Verification items for the finished model (mm, model axes). A direction names the side the tool comes from. Coordinates: 2 decimals unless noted, no trailing zeros. Write each loop counter-clockwise with the first axis right and the second up, starting at its lowest first coordinate (ties: lowest second). Pieces come first, ordered by that corner, then holes. Notation, with made-up numbers: (-22, 61.25) -> (-16, 61.25) arc R24 cw to (-16, 94.25) -> close; hole circle Ø1 at (36.5, 40.25). An arc over 180 degrees is marked (long way). Use a Markdown table: item, result. Add a question column.
Autodesk Inventor part; units mm, degrees
ref_plane "YZ Plane" through (0, 0, 0) normal (1, 0, 0) x (0, 1, 0)
ref_plane "XZ Plane" through (0, 0, 0) normal (0, 1, 0) x (-1, 0, 0)
ref_plane "XY Plane" through (0, 0, 0) normal (0, 0, 1) x (1, 0, 0)
sketch "Sketch1" plane through (0, 0, 0) normal (0, 0, 1) x (1, 0, 0)
  line L0 (-110, 70) -> (110, 70) construction
  line L1 (110, 70) -> (110, -70) construction
  line L2 (110, -70) -> (-110, -70) construction
  line L3 (-110, -70) -> (-110, 70) construction
  circle A0 centre (-90, 55) radius 5
  circle A1 centre (-90, -55) radius 5
  circle A2 centre (90, -55) radius 5
  circle A3 centre (-10, 45) radius 5
  line L4 (-67, 0) -> (-42, 0) construction
  line L5 (-42, 0) -> (-42, -30) construction
  line L6 (-42, -30) -> (-67, -30) construction
  line L7 (-67, -30) -> (-67, 0) construction
  circle A4 centre (-54.5, -11) radius 10 construction
  circle A5 centre (-63.5044, -24.4163) radius 3 construction
  circle A6 centre (-57.3559, -26.4695) radius 3 construction
  circle A7 centre (-51.263, -24.6531) radius 3 construction
  circle A8 centre (-45.3418, -26.5938) radius 3 construction
  arc A9 (-75, 54.9997) -> (-105, 55) centre (-90, 55) ccw
  arc A10 (-105, -55) -> (-90, -70) centre (-90, -55) ccw
  line L8 (-105, 55) -> (-105, -55)
  line L9 (-67.173, 37.0938) -> (-15.8457, 58.814)
  arc A11 (-80.9053, 10.3283) -> (-28.4795, 28.932) centre (-131.69, 236.6113) ccw
  arc A12 (-84.9945, -37.6763) -> (-83.834, 6.647) centre (-774.2501, 2.5469) ccw
  arc A13 (-74.1138, 41.4213) -> (-75, 54.9997) centre (-774.2501, 2.5469) ccw
  arc A14 (-74.1138, 41.4213) -> (-67.173, 37.0938) centre (-69.1215, 41.6985) ccw
  arc A15 (-80.9053, 10.3283) -> (-83.834, 6.647) centre (-80.0841, 6.6693) ccw
  arc A16 (-84.9945, -37.6763) -> (-79.3208, -42.9208) centre (-80.003, -37.9675) ccw
  arc A17 (-0.2374, 33.6118) -> (-15.8457, 58.814) centre (-10, 45) ccw
  arc A18 (87.1375, -69.7243) -> (81.0789, -42.9413) centre (90, -55) ccw
  arc A19 (90, -70) -> (-90, -70) centre (0, -989.5783) ccw
  line L10 (5, 45) -> (5, -37.2895)
  arc A20 (-21.304, 23.7513) -> (-20.2259, -37.0973) centre (169.1855, -3.3075) ccw
  line L11 (-19.6904, 33.6118) -> (-19.6904, -39.9724) construction
  line L12 (-19.6904, 33.6118) -> (53.8938, 33.6118) construction
  arc A21 (-21.304, 23.7513) -> (-28.4795, 28.932) centre (-26.2543, 24.4545) ccw
  arc A22 (-22.6296, -40.0357) -> (-20.2259, -37.0973) centre (-22.687, -37.5364) ccw
  arc A23 (5, -37.2895) -> (7.4835, -39.7895) centre (7.5, -37.2895) ccw
  arc A24 (81.0789, -42.9413) -> (7.4835, -39.7895) centre (0.7495, -1057.8516) ccw
  arc A25 (-22.6296, -40.0357) -> (-79.3208, -42.9208) centre (0.7495, -1057.8516) ccw
  point P0 (0, 0)
  point P1 (90, -70)
  dimension "d1" = 70
  dimension "d2" = 70
  dimension "d3" = 110
  dimension "d4" = 110
  dimension "d5" = 10
  dimension "d6" = 10
  dimension "d7" = 10
  dimension "d8" = 10
  dimension "d9" = 55
  dimension "d10" = 55
  dimension "d11" = 55
  dimension "d12" = 180
  dimension "d13" = 90
  dimension "d14" = 90
  dimension "d15" = 10
  dimension "d16" = 45
  dimension "d17" = 42
  dimension "d18" = 30
  dimension "d19" = 0
  dimension "d20" = 25
  dimension "d21" = 20
  dimension "d22" = 6
  dimension "d23" = 6
  dimension "d24" = 6
  dimension "d25" = 11
  dimension "d26" = 12.5
  dimension "d27" = 6
  dimension "d50" = 30
  dimension "d51" = 30
  dimension "d53" = 10
  dimension "d54" = 7.5
  dimension "d58" = 10
  dimension "d59" = 30
  dimension "d60" = 30
  dimension "d61" = 90
  dimension "d62" = 10
  dimension "d63" = 5
  dimension "d64" = 5
extrude "Extrusion5" add sketch "Sketch1" along normal blind 9.4 contours A13 A14 L9 A17 L10 A23 A24 A18 A19 A10 L8 A9
equation "\"d26\" = 0.5 * d20"
properties part number "Bracket Concept MK7"
1) Gauge pin test, flat ends, axial feed: pin 1 (2 mm diameter, centred on x = -44, z = 1, fed in from +Y); pin 2 (3 mm diameter, centred on y = -3, z = 6, fed in from +X); pin 3 (6 mm diameter, centred on x = -90, y = 55, fed in from +Z); pin 4 (3 mm diameter, centred on x = -18, z = 4.5, fed in from +Y). Record the tip position at first contact, or that the pin passes through.
2) Cross-section at D-D on x = 79. Record the boundary of the cut face in (y, z), then the cut area to 3 significant figures.
3) Cross-section at B-B on x = -10. Record the boundary of the cut face in (y, z).
4) Thickness scan on L1, parallel to Y at x = -90, z = 3.25; L2, parallel to X at y = 40.5, z = 1.5; L3, parallel to X at y = -20.5, z = 4.75. Record the ranges inside material, lowest first.
5) Cross-section at C-C on z = 2.5. Record the boundary of the cut face in (x, y), then the cut area to 3 significant figures.
6) Set-up check for faces 1 (the face through (-23.18, -7.14, 4.63)), 2 (the face through (43.794, -40.678, 4.634)), 3 (the face through (-1, -15, 0)): record each of +Z, -Z, +X, -X, +Y, -Y from which the full face is reachable in a straight line by a thin tool's end or side.
7) Cross-section at A-A on y = -20.5. Record the boundary of the cut face in (x, z).
8) Release check for a two-part mould opening along X. For faces 4 (the face through (5, 4, 5)), 5 (the face through (-105, 1, 5)), 6 (the face through (-41.87, 47.8, 4.63)) record: released by +X, released by -X, zero draft, split by the parting line, or undercut.
Returned:
| question | item | result |
|---|---|---|
| 1 | pin 1 | stops at y = 47.32 |
| 1 | pin 2 | stops at x = 5 |
| 1 | pin 3 | passes through |
| 1 | pin 4 | stops at y = 58.54 |
| 2 | outline | (-68.99, 0) -> (-42.78, 0) -> (-42.78, 9.4) -> (-68.99, 9.4) -> close |
| 2 | area | 246 mm² |
| 3 | outline | (-65.66, 0) -> (40, 0) -> (40, 9.4) -> (-65.66, 9.4) -> close; (50, 0) -> (60, 0) -> (60, 9.4) -> (50, 9.4) -> close |
| 4 | L1 | y = -70 to -60, -50 to 50, 60 to 70 |
| 4 | L2 | x = -105 to -73.98, -59.12 to -12.18, -7.82 to 5 |
| 4 | L3 | x = -105 to -84.21, -22.45 to 5 |
| 5 | outline | (-105, -55) arc R15 ccw to (-90, -70) arc R923.97 cw to (90, -70) arc R15 ccw (long way) to (81.08, -42.94) arc R1018.11 ccw to (7.48, -39.79) arc R2.5 cw to (5, -37.29) -> (5, 45) arc R15 ccw to (-15.85, 58.81) -> (-67.17, 37.09) arc R5 cw to (-74.11, 41.42) arc R700.77 ccw to (-75, 55) arc R15 ccw to (-105, 55) -> close; hole circle Ø10 at (-90, -55); hole circle Ø10 at (-90, 55); hole (-84.99, -37.68) arc R5 ccw to (-79.32, -42.92) arc R1018.08 cw to (-22.63, -40.04) arc R2.5 ccw to (-20.23, -37.1) arc R192.4 cw to (-21.3, 23.75) arc R5 ccw to (-28.48, 28.93) arc R231.91 cw to (-80.91, 10.33) arc R3.75 ccw to (-83.83, 6.65) arc R690.44 cw to start; hole circle Ø10 at (-10, 45); hole circle Ø10 at (90, -55) |
| 5 | area | 11,900 mm² |
| 6 | face 1 | +Z, -Z |
| 6 | face 2 | +Z, -Z, +Y |
| 6 | face 3 | -Z, +X, -X, +Y, -Y |
| 7 | outline | (-105, 0) -> (-84.21, 0) -> (-84.21, 9.4) -> (-105, 9.4) -> close; (-22.45, 0) -> (5, 0) -> (5, 9.4) -> (-22.45, 9.4) -> close |
| 8 | face 4 | released by +X |
| 8 | face 5 | released by -X |
| 8 | face 6 | undercut |
